```python
from build123d import *

# Parameters (mm, degrees)
EXTRUDE_2_DEPTH     = 4
EXTRUDE_3_DEPTH     = 51.85
EXTRUDE_4_DEPTH     = 51.85
SKETCH_6_W          = 25
SKETCH_6_H          = 12
CUT_EXTRUDE_1_DEPTH = 4
SKETCH_7_W          = 46
SKETCH_7_H          = 4
EXTRUDE_5_DEPTH     = 1.15
EXTRUDE_6_DEPTH     = 5
EXTRUDE_7_DEPTH     = 1
FILLET_3_R          = 2


with BuildPart() as part:
    # 草图1 → 凸台-拉伸2 (new body)
    with BuildSketch(Plane(origin=(0, 0, 0), x_dir=(1, 0, 0), z_dir=(0, 1, 0))):
        Polygon((16.85, -20.85), (17, -20.85), (17, 20.85), (16.85, 20.85), (-34.85, 20.85), (-34.85, -20.85), align=None)
        Polygon((17, -20.85), (17, -21), (31, -21), (35, -21), (35, -18), (35, 18), (35, 21), (31, 21), (17, 21), (17, 20.85), align=None)
        Polygon((31, -21), (17, -21), (17, -23), (37, -23), (37, 23), (17, 23), (17, 21), (31, 21), (35, 21), (35, 18), (35, -18), (35, -21), align=None)
    extrude(amount=EXTRUDE_2_DEPTH)

    # 草图4 → 凸台-拉伸3 (add)
    with BuildSketch(Plane.ZY.offset(-17)):
        Polygon((-20.85, 2), (-21.85, 1), (-20.85, 0), align=None)
    extrude(amount=EXTRUDE_3_DEPTH)

    # 草图3 → 凸台-拉伸4 (add)
    with BuildSketch(Plane.ZY.offset(-17)):
        Polygon((20.85, 2), (21.85, 1), (20.85, 0), align=None)
    extrude(amount=EXTRUDE_4_DEPTH)

    # 草图6 → 切除-拉伸1 (cut)
    with BuildSketch(Plane(origin=(0, 4, 0), x_dir=(1, 0, 0), z_dir=(0, 1, 0))):
        with Locations((-19.35, -0.15)):
            Rectangle(SKETCH_6_W, SKETCH_6_H)
    extrude(amount=-CUT_EXTRUDE_1_DEPTH, mode=Mode.SUBTRACT)

    # 草图7 → 凸台-拉伸5 (add)
    with BuildSketch(Plane(origin=(37, 0, 0), x_dir=(0, 0, -1), z_dir=(1, 0, 0))):
        with Locations((0, 2)):
            Rectangle(SKETCH_7_W, SKETCH_7_H)
    extrude(amount=EXTRUDE_5_DEPTH)

    # 草图12 → 凸台-拉伸6 (add, symmetric)
    with BuildSketch(Plane.XY):
        Polygon((36.65, 0), (36.65, -0.75), (37.4, 0), align=None)
        Polygon((35.9, 0), (36.65, -0.75), (36.65, 0), align=None)
    extrude(amount=EXTRUDE_6_DEPTH, both=True)

    # 草图14 → 凸台-拉伸7 (add)
    with BuildSketch(Plane.ZY.offset(34.85)):
        Polygon((-20.85, 0), (20.85, 0), (21.85, 1), (20.85, 2), (20.85, 4), (-20.85, 4), (-20.85, 2), (-21.85, 1), align=None)
    extrude(amount=EXTRUDE_7_DEPTH)

    # 圆角3
    fillet_3_edges = [part.edges().sort_by_distance(p)[0] for p in [
        (27.575, 4, 23),
        (27.575, 4, -23),
        (38.15, 2, 23),
        (38.15, 2, -23),
        (38.15, 4, 0),
    ]]
    fillet(fillet_3_edges, radius=FILLET_3_R)


solid = part.part
```
Read the model definition and answer for the solid it produces. Units are mm, in the model's axes. A direction names the side the tool comes from. Give positions to 0.01 mm unless a question says otherwise; leave off trailing zeros. Loops run counter-clockwise (first coordinate to the right, second up) from the corner with the lowest first, then second, coordinate; pieces in that order, holes last.
Item 1: The mould has two halves that part along Z. Classify faces 1 (the flat face through (2, 0, 0)), 2 (the flat face through (-20, 2, -5.85)), 3 (the cylindrical face through (37.58, 1.01, 22.4)): released by +Z, released by -Z, zero draft, split by the parting line, or undercut.
Item 2: For faces 4 (the flat face through (-31.85, 2, 0)), 5 (the flat face through (-9, 3, -20.85)), 6 (the flat face through (-9, 3, 20.85)), determine the directions among +Z, -Z, +X, -X, +Y, -Y from which every point of the face is accessible in a straight line to the end or side of a thin tool.
Item 3: The part is cut by section A-A (x = -29). Write down the section's boundary in (y, z).
Item 4: The part is cut by section C-C (x = 12). Write down the section's boundary in (y, z).
Item 5: Find the intervals of material crossed by line 1 along X through (y, z) = (0.45, -5.5); line 2 along Z through (x, y) = (-20.5, 2.25); line 3 along Y through (x, z) = (7, -2.5), in increasing order.
Item 6: Each of these flat-tipped pins is pushed along its axis until it touches: pin 1 Ø1.1 at (y, z) = (2.5, 22) entering from -X; pin 2 Ø4 at (x, z) = (4, 2.5) entering from -Y; pin 3 Ø1.6 at (x, y) = (-22.5, 2.5) entering from +Z. Where does it stop, or does it pass through?
Item 7: The part is cut by section B-B (z = 2). Write down the section's boundary in (x, y).
Item 8: The part is cut by section D-D (y = 3.3). Write down the section's boundary in (x, z), and give its area (3 significant figures).
Taken from the geometry:
1. face 1: zero draft
1. face 2: undercut
1. face 3: released by +Z
2. face 4: +Y, -Y
2. face 5: -Z, -X, +Y
2. face 6: +Z, -X, +Y
3. outline: (0, -20.85) - (1, -21.85) - (2, -20.85) - (4, -20.85) - (4, -5.85) - (0, -5.85) - close; (0, 6.15) - (4, 6.15) - (4, 20.85) - (2, 20.85) - (1, 21.85) - (0, 20.85) - close
4. outline: (0, -20.85) - (1, -21.85) - (2, -20.85) - (4, -20.85) - (4, 20.85) - (2, 20.85) - (1, 21.85) - (0, 20.85) - close
5. line 1: x = -35.85 to -31.85, -6.85 to 38.15
5. line 2: z = -20.85 to -5.85, 6.15 to 20.85
5. line 3: y = 0 to 4
6. pin 1: stops at x = 17
6. pin 2: stops at y = 0
6. pin 3: stops at z = 21.15
7. outline: (-35.85, 0) - (-31.85, 0) - (-31.85, 4) - (-35.85, 4) - close; (-6.85, 0) - (35.9, 0) - (36.65, -0.75) - (37.4, 0) - (38.15, 0) - (38.15, 2) arc R2 ccw to (36.15, 4) - (-6.85, 4) - close
8. outline: (-35.85, -20.85) - (17, -20.85) - (17, -22.52) - (36.15, -22.52) arc R1.52 ccw to (37.67, -21) - (37.67, 21) arc R1.52 ccw to (36.15, 22.52) - (17, 22.52) - (17, 20.85) - (-35.85, 20.85) - close; hole (-31.85, -5.85) - (-6.85, -5.85) - (-6.85, 6.15) - (-31.85, 6.15) - close
8. area: 2,830 mm2
